Input: part model. Units: mm. Frame: model coordinates. Face numbers are marked on the shaded views. A direction names the side the tool comes from. Round coordinates to 2 decimals unless told otherwise and drop trailing zeros. Loops run counter-clockwise (first coordinate to the right, second up) from the corner with the lowest first, then second, coordinate; pieces in that order, holes last. Notation, with made-up numbers: (-16.75, -3.75) - (1.25, -3.75) arc R26 ccw to (1.25, 30.25) - close; hole circle Ø10 at (15, 87.25). An arc over 180 degrees is marked (long way). Write each question's results on one line, items separated by ' | '.
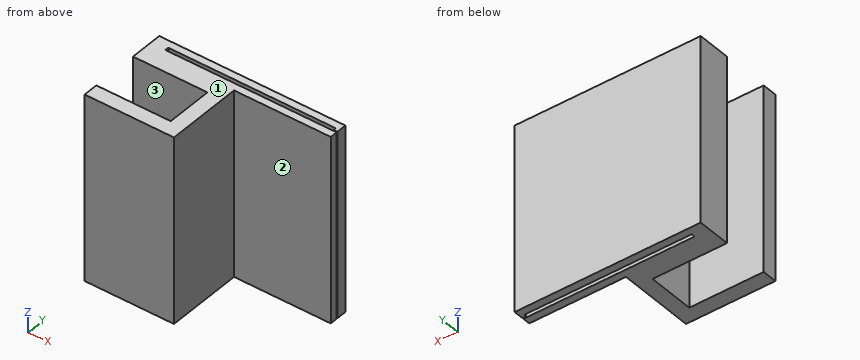
from build123d import *

# Parameters (mm, degrees)
F0_W     = 2
F0_H     = 0.5
F0_H_2   = 6.3
F0_W_2   = 0.5
F0_H_3   = 0.35
F1_DEPTH = 25


with BuildPart() as f1:
    # F0 (on Top) → F1 (new body)
    with BuildSketch(Plane.XY):
        Polygon((-10, 6.15), (-10, 5.15), (2, 5.15), (15, 5.15), (15, 6.15), (-8, 6.15), align=None)
        Polygon((2, 5.15), (-10, 5.15), (-10, 3.15), (0, 3.15), (2, 3.15), align=None)
        with Locations((-9, 6.4)):
            Rectangle(F0_W, F0_H)
        with Locations((1, 0)):
            Rectangle(F0_W, F0_H_2)
        Polygon((-10, 7.65), (-10, 6.65), (-8, 6.65), (14.5, 6.65), (15, 6.65), (15, 7.65), align=None)
        Polygon((2, -5.15), (2, -3.15), (0, -3.15), (-10, -3.15), (-10, -5.15), align=None)
        with Locations((14.75, 6.475)):
            Rectangle(F0_W_2, F0_H_3)
    extrude(amount=F1_DEPTH)


solid = f1.part
1. Section query D-D, the plane y = -1. Output: boundary loops of the cut face in (x, z), plus the area to 3 significant figures.
Answer:
outline: (0, 0) - (2, 0) - (2, 25) - (0, 25) - close | area: 50.0 mm^2
2. Section query A-A, the plane x = 2.5. Output: boundary loops of the cut face in (y, z).
Answer:
outline: (5.15, 0) - (6.15, 0) - (6.15, 25) - (5.15, 25) - close; (6.65, 0) - (7.65, 0) - (7.65, 25) - (6.65, 25) - close
3. Contact query for flat-ended pins moving along their axis: pin 1 (0.6 mm diameter, centred on x = 15, z = 18, fed in from -Y); pin 2 (1 mm diameter, centred on y = 4, z = 22, fed in from +X). Output: stop coordinate, or through.
Answer:
pin 1: y = 5.15 | pin 2: x = 2
4. Section query C-C, the plane z = 14. Output: boundary loops of the cut face in (x, y), plus the area to 3 significant figures.
Answer:
outline: (-10, -5.15) - (2, -5.15) - (2, 5.15) - (15, 5.15) - (15, 6.15) - (-8, 6.15) - (-8, 6.65) - (14.5, 6.65) - (14.5, 6.3) - (15, 6.3) - (15, 7.65) - (-10, 7.65) - (-10, 3.15) - (0, 3.15) - (0, -3.15) - (-10, -3.15) - close | area: 112 mm^2
5. Section query B-B, the plane x = -6. Output: boundary loops of the cut face in (y, z).
Answer:
outline: (-5.15, 0) - (-3.15, 0) - (-3.15, 25) - (-5.15, 25) - close; (3.15, 0) - (6.15, 0) - (6.15, 25) - (3.15, 25) - close; (6.65, 0) - (7.65, 0) - (7.65, 25) - (6.65, 25) - close
6. Line query: line 1 (Y direction, x = -1.25, z = 2.75); line 2 (Y direction, x = 11.5, z = 17); line 3 (Y direction, x = 0.25, z = 16.5). Output: solid intervals per line, ascending. Write a range as [from, to].
Answer:
line 1: [-5.15, -3.15], [3.15, 6.15], [6.65, 7.65] | line 2: [5.15, 6.15], [6.65, 7.65] | line 3: [-5.15, 6.15], [6.65, 7.65]
7. Set-up query: the marked faces 1, 2 and 3. Return all of +Z, -Z, +X, -X, +Y, -Y with unobstructed straight access to the full face (end or side cutting, diameter ignored); none if empty.
Answer:
face 1: +Z, +X, -X, +Y, -Y | face 2: +Z, -Z, +X, -Y | face 3: +Z, -Z, -X
